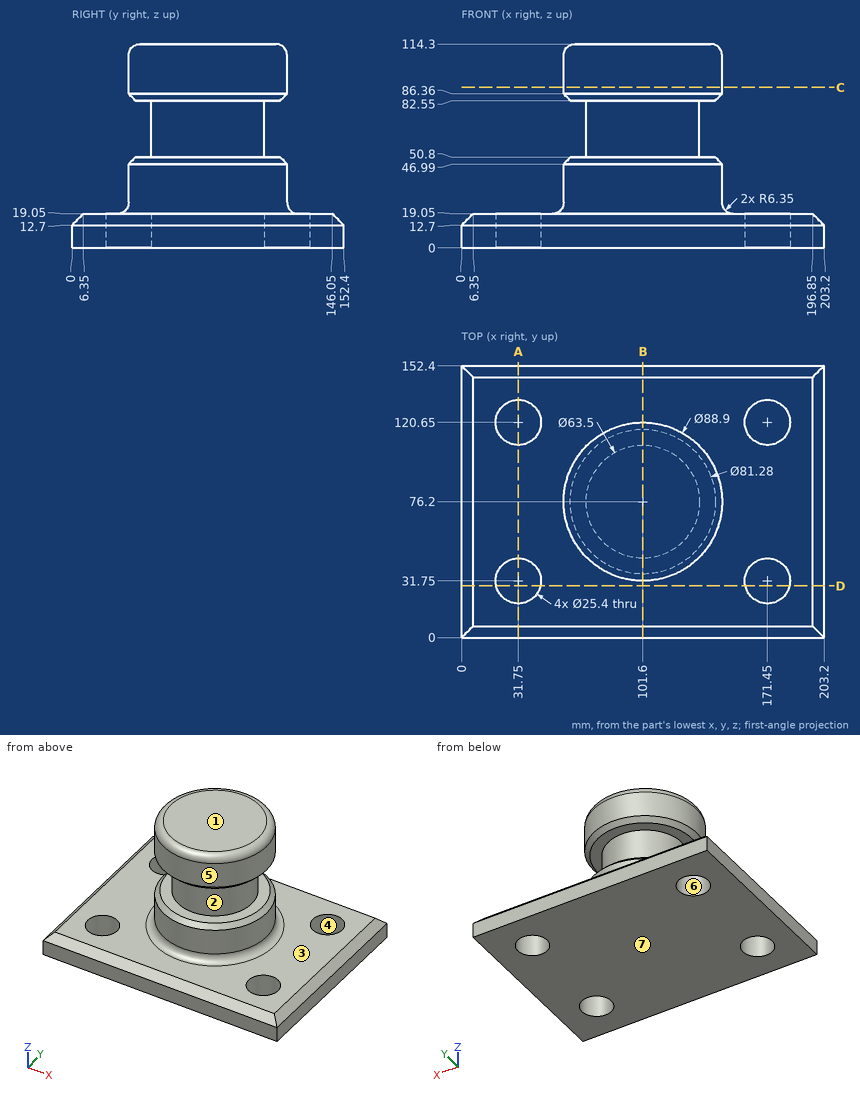
Verification items for this drawing (mm, ordinates from the low corner). A direction names the side the tool comes from. Coordinates: 2 decimals unless noted, no trailing zeros. Order: outer loops, then holes, each group sorted by start corner. A loop starts at its lowest first (then second) coordinate and runs counter-clockwise, first axis right, second up. Notation, with made-up numbers: (45.25, 34) - (61.25, 34) arc R18 cw to (61.25, 62) - close; hole circle Ø10 at (15.5, 39.25). An arc over 180 degrees is marked (long way). Answer as a JSON object with one key per item and string values. Group by question number.
Item 1: Sectioned sample at D-D, the plane y = 29. Give the number of separate pieces and of enclosed holes in the cut face, and give its area (3 significant figures).
Item 2: Sectioned sample at C-C, the plane z = 90. Record the cut outline in (x, y), and give its area (3 significant figures).
Item 3: Sectioned sample at A-A, the plane x = 31.75. Record the cut outline in (y, z).
Item 4: Tool access check on the marked faces 1, 2 and 3. Record the directions out of +Z, -Z, +X, -X, +Y, -Y that give a thin tool (end or side, any length) a straight path to the whole face; none if there is none.
Item 5: Draft check along Y on the marked faces 4, 5, 6 and 7. Enter one of: +Y half, -Y half, draft (parallel to the pull), parting line (faces both ways), or undercut.
Item 6: Depth check by flat-ended pin: pin 1 Ø1.5 at (y, z) = (56.5, 76.5) entering from -X; pin 2 Ø5 at (y, z) = (80.5, 67.5) entering from -X; pin 3 Ø8 at (x, z) = (114.5, 42) entering from -Y. Enter the tip coordinate at first touch or a pass-through.
Item 7: Sectioned sample at B-B, the plane x = 101.6. Record the cut outline in (y, z).
Item 8: Scan lines: probe 1 along Y at (x, z) = (171.45, 10.75); probe 2 along X at (y, z) = (31, 9); probe 3 along Y at (x, z) = (31, 13). Record each from-to range of solid material in increasing order.
Resolved:
{
 "1": {"separate pieces": "3", "enclosed holes": "0", "area": "2,910 mm^2"},
 "2": {"outline": "circle Ø88.9 at (101.6, 76.2)", "area": "6,210 mm^2"},
 "3": {"outline": "(0, 0) - (19.05, 0) - (19.05, 19.05) - (6.35, 19.05) - (0, 12.7) - close; (44.45, 0) - (107.95, 0) - (107.95, 19.05) - (44.45, 19.05) - close; (133.35, 0) - (152.4, 0) - (152.4, 12.7) - (146.05, 19.05) - (133.35, 19.05) - close"},
 "4": {"face 1": "+Z, +X, -X, +Y, -Y", "face 2": "none", "face 3": "+Z"},
 "5": {"face 4": "undercut", "face 5": "parting line", "face 6": "undercut", "face 7": "draft"},
 "6": {"pin 1": "x = 76.13", "pin 2": "x = 69.9", "pin 3": "y = 32.65"},
 "7": {"outline": "(0, 0) - (152.4, 0) - (152.4, 12.7) - (146.05, 19.05) - (127, 19.05) arc R6.35 cw to (120.65, 25.4) - (120.65, 46.99) - (116.84, 50.8) - (107.95, 50.8) - (107.95, 82.55) - (116.84, 82.55) - (120.65, 86.36) - (120.65, 107.95) arc R6.35 ccw to (114.3, 114.3) - (38.1, 114.3) arc R6.35 ccw to (31.75, 107.95) - (31.75, 86.36) - (35.56, 82.55) - (44.45, 82.55) - (44.45, 50.8) - (35.56, 50.8) - (31.75, 46.99) - (31.75, 25.4) arc R6.35 cw to (25.4, 19.05) - (6.35, 19.05) - (0, 12.7) - close"},
 "8": {"probe 1": "0 to 19.05, 44.45 to 107.95, 133.35 to 152.4", "probe 2": "0 to 19.07, 44.43 to 158.77, 184.13 to 203.2", "probe 3": "0.3 to 19.07, 44.43 to 107.97, 133.33 to 152.1"}
}
